```python
from build123d import *

# Parameters (mm, degrees)
SKETCH1_R           = 35
BOSS_EXTRUDE1_DEPTH = 30
SKETCH2_R           = 34.3
CUT_EXTRUDE1_DEPTH  = 25
FILLET1_R           = 1
FILLET2_R           = 0.2


with BuildPart() as part:
    # Sketch1 → Boss-Extrude1 (new body)
    with BuildSketch(Plane(origin=(0, 0, 0), x_dir=(1, 0, 0), z_dir=(0, 1, 0))):
        Circle(SKETCH1_R)
    extrude(amount=BOSS_EXTRUDE1_DEPTH)

    # Sketch2 → Cut-Extrude1 (cut)
    with BuildSketch(Plane(origin=(0, 0, 0), x_dir=(1, 0, 0), z_dir=(0, 1, 0))):
        Circle(SKETCH2_R)
    extrude(amount=CUT_EXTRUDE1_DEPTH, mode=Mode.SUBTRACT)

    # Fillet1
    fillet1_edges = [part.edges().sort_by_distance(p)[0] for p in [
        (-35, 30, 0),
    ]]
    fillet(fillet1_edges, radius=FILLET1_R)

    # Fillet2
    fillet2_edges = [part.edges().sort_by_distance(p)[0] for p in [
        (-35, 0, 0),
    ]]
    fillet(fillet2_edges, radius=FILLET2_R)


solid = part.part
```
The listing builds one solid part. Answer for the finished solid, in the listing's coordinates (mm). A direction names the side the tool comes from. Give positions to 0.01 mm unless a question says otherwise; leave off trailing zeros. Write each loop counter-clockwise with the first axis right and the second up, starting at its lowest first coordinate (ties: lowest second). Pieces come first, ordered by that corner, then holes. Notation, with made-up numbers: (85, -38) -> (125, -38) arc R23 cw to (125, -8) -> close; hole circle Ø2 at (54, 75.5). An arc over 180 degrees is marked (long way). Use one line per item in the form item = value.
1) Straight lines are drawn through the part: probe 1 along X at (y, z) = (17.5, 0); probe 2 along Y at (x, z) = (23.5, 10). For each, find the intervals that lie inside material, in ascending order.
Result:
probe_1 = -35 to -34.3, 34.3 to 35
probe_2 = 25 to 30
2) A tool of negligible diameter and unlimited length cuts with its end or side. For faces 4 (the flat face through (0, 30, 0)), 5 (the flat face through (0, 25, 0)), from which of +Z, -Z, +X, -X, +Y, -Y can it reach the whole face along a straight path? Write none if from no direction.
Result:
face_4 = +Z, -Z, +X, -X, +Y
face_5 = -Y
3) For a pull along X with two mould halves and no side action, classify faces 1 (the cylindrical face through (-28, 14, 21)), 2 (the flat face through (25.62, 0, 23.04)), 3 (the cylindrical face through (32.716, 12.325, -10.303)) as +X half, -X half, draft (parallel to the pull), parting line (faces both ways), or undercut.
Result:
face_1 = parting line
face_2 = draft
face_3 = undercut
4) Section A-A on x = 0 is taken. Write down the section's boundary in (y, z), plus the area to 3 significant figures.
Result:
outline = (0, -34.8) arc R0.2 ccw to (0.2, -35) -> (29, -35) arc R1 ccw to (30, -34) -> (30, 34) arc R1 ccw to (29, 35) -> (0.2, 35) arc R0.2 ccw to (0, 34.8) -> (0, 34.3) -> (25, 34.3) -> (25, -34.3) -> (0, -34.3) -> close
area = 385 mm²
5) Each of these flat-tipped pins is pushed along its axis until it touches: P1, Ø8, axis at x = 23.5, y = 10.5, coming from the -Z side; P2, Ø5, axis at x = -2, z = 20, coming from the -Y side; P3, Ø5, axis at y = 16, z = 14.5, coming from the +X side. Where does it stop, or does it pass through?
Result:
P1 = -29.06
P2 = 25
P3 = 32.88
6) Section C-C on y = 21.25 is taken. Write down the section's boundary in (x, z).
Result:
outline = circle Ø70 at (0, 0); hole circle Ø68.6 at (0, 0)
7) Section B-B on z = 0 is taken. Write down the section's boundary in (x, y).
Result:
outline = (-35, 0.2) arc R0.2 ccw to (-34.8, 0) -> (-34.3, 0) -> (-34.3, 25) -> (34.3, 25) -> (34.3, 0) -> (34.8, 0) arc R0.2 ccw to (35, 0.2) -> (35, 29) arc R1 ccw to (34, 30) -> (-34, 30) arc R1 ccw to (-35, 29) -> close
8) Section D-D on y = 26.75 is taken. Write down the section's boundary in (x, z).
Result:
outline = circle Ø70 at (0, 0)
